from build123d import *

# Parameters (mm, degrees)
BOX003_W                    = 10
BOX003_H                    = 10
BOX003_DEPTH                = 10
CYLINDER002_R               = 1.8
CYLINDER002_DEPTH           = 9
BOX030_W                    = 1
BOX030_H                    = 2
BOX030_DEPTH                = 9
CYLINDER010_R               = 3
CYLINDER010_DEPTH           = 9
CYLINDER012_W               = 20
CYLINDER012_H               = 10
CYLINDER012_ANGLE           = 70
CYLINDER012_PLACEMENT_ANGLE = 235
ARRAY_COUNT                 = 5
TORUS_R                     = 1.5
CYLINDER_R                  = 25
CYLINDER_DEPTH              = 5
CUT024_ROLL_ANGLE           = 90
CUT024_PLACEMENT_ANGLE      = 180


with BuildPart() as cube002:
    # Box003 → Box003 (new body)
    with BuildSketch(Plane(origin=(-3, 1.1, 0), x_dir=(1, 0, 0), z_dir=(0, 0, 1))):
        with Locations((5, 5)):
            Rectangle(BOX003_W, BOX003_H)
    extrude(amount=BOX003_DEPTH)


with BuildPart() as shafthole:
    # Cylinder002 → Cylinder002 (new body)
    with BuildSketch(Plane.XY):
        Circle(CYLINDER002_R)
    extrude(amount=CYLINDER002_DEPTH)

    # Cut002: cut Cube002
    add(cube002.part, mode=Mode.SUBTRACT)


with BuildPart() as fusion015:
    # Box030 → Box030 (new body)
    with BuildSketch(Plane(origin=(-0.5, -3.5, 0), x_dir=(1, 0, 0), z_dir=(0, 0, 1))):
        with Locations((0.5, 1)):
            Rectangle(BOX030_W, BOX030_H)
    extrude(amount=BOX030_DEPTH)

    # Fusion015: union shaftHole
    add(shafthole.part)


with BuildPart() as cylinder010:
    # Cylinder010 → Cylinder010 (new body)
    with BuildSketch(Plane.XY):
        Circle(CYLINDER010_R)
    extrude(amount=CYLINDER010_DEPTH)


with BuildPart() as array022:
    # Cylinder012 → Cylinder012 (revolve)
    with BuildSketch(Plane.XZ):
        with Locations((10, 5)):
            Rectangle(CYLINDER012_W, CYLINDER012_H)
    revolve(axis=Axis((0, 0, 0), (0, 0, 1)), revolution_arc=CYLINDER012_ANGLE)


with BuildPart() as array022_1:
    # Cylinder012 placement: moved
    add(array022.part.moved(Location((0, -2, 0))).rotate(Axis((0, -2, 0), (0, 0, 1)), CYLINDER012_PLACEMENT_ANGLE))

    # Array: Array022 ×5 about axis
    array_axis = Axis((0, 0, 0), (0, 0, 1))


with BuildPart() as array022_2:
    add(array022_1.part)
    for i in range(1, ARRAY_COUNT):
        add(array022_1.part.rotate(array_axis, i * 360 / ARRAY_COUNT))


with BuildPart() as torus:
    # Torus → Torus (revolve)
    with BuildSketch(Plane(origin=(0, 0, 2.5), x_dir=(1, 0, 0), z_dir=(0, -1, 0))):
        with Locations((25, 0)):
            Circle(TORUS_R)
    revolve(axis=Axis((0, 0, 2.5), (0, 0, 1)))


with BuildPart() as wheel:
    # Cylinder → Cylinder (new body)
    with BuildSketch(Plane.XY):
        Circle(CYLINDER_R)
    extrude(amount=CYLINDER_DEPTH)

    # Cut001: cut Torus
    add(torus.part, mode=Mode.SUBTRACT)

    # Cut023: cut Array022
    add(array022_2.part, mode=Mode.SUBTRACT)

    # Fusion016: union Cylinder010
    add(cylinder010.part)

    # Cut024: cut Fusion015
    add(fusion015.part, mode=Mode.SUBTRACT)


with BuildPart() as wheel_1:
    # Cut024 roll: moved
    add(wheel.part.rotate(Axis((0, 0, 0), (1, 0, 0)), CUT024_ROLL_ANGLE))


with BuildPart() as wheel_2:
    # Cut024 placement: moved
    add(wheel_1.part.moved(Location((-10.9, -46, 9.8))).rotate(Axis((-10.9, -46, 9.8), (0, 0, 1)), CUT024_PLACEMENT_ANGLE))


solid = wheel_2.part
Model file for the job. Use its own axes, mm. Coordinates: 2 decimals unless noted, no trailing zeros. Write each question's results on one line, items separated by ' | '. Start each with the question number.
1) Mould opens along Z. For faces 1 (the face through (-19.08, -43.46, 0.85)), 2 (the face through (-22.4, -41.5, -12.4)), 3 (the face through (-9, -46, 8)) say: pulls with the +Z half, pulls with the -Z half, needs draft (parallel to the pull), parting line crosses it, or undercut.
2) Probe line 1 along Z through (x, y) = (-8.5, -43); line 2 along Z through (x, y) = (0, -44.75); line 3 along X through (y, z) = (-44, -2.5). List the from-to ranges inside material, lowest first. Write a range as from..to.
3) Cut at A-A (x = -6.5). Count the separate pieces of the cut face and the enclosed holes in it, then the cut area to 3 significant figures.
4) Flat gauge pins, fed straight in: P1, Ø1, axis at y = -41.5, z = 18.5, coming from the -X side; P2, Ø1.4, axis at y = -41, z = 7.5, coming from the -X side; P3, Ø5, axis at y = -44, z = 7, coming from the +X side. Where does each tip first touch, or does it go through?
Returned:
1) face 1: undercut | face 2: parting line crosses it | face 3: needs draft
2) line 1: -13.66..-12.06, 4.37..11.84, 31.38..33.26 | line 2: -11.77..-8.97, -7.77..-2.76, 11.93..14.77, 28.89..31.37 | line 3: -31.02..-29.04, -21.61..-18.11, -3.69..-0.19, 7.24..9.22
3) separate pieces: 4 | enclosed holes: 0 | area: 59.2 mm^2
4) P1: x = -34.52 | P2: x = -35.85 | P3: x = 14.09
